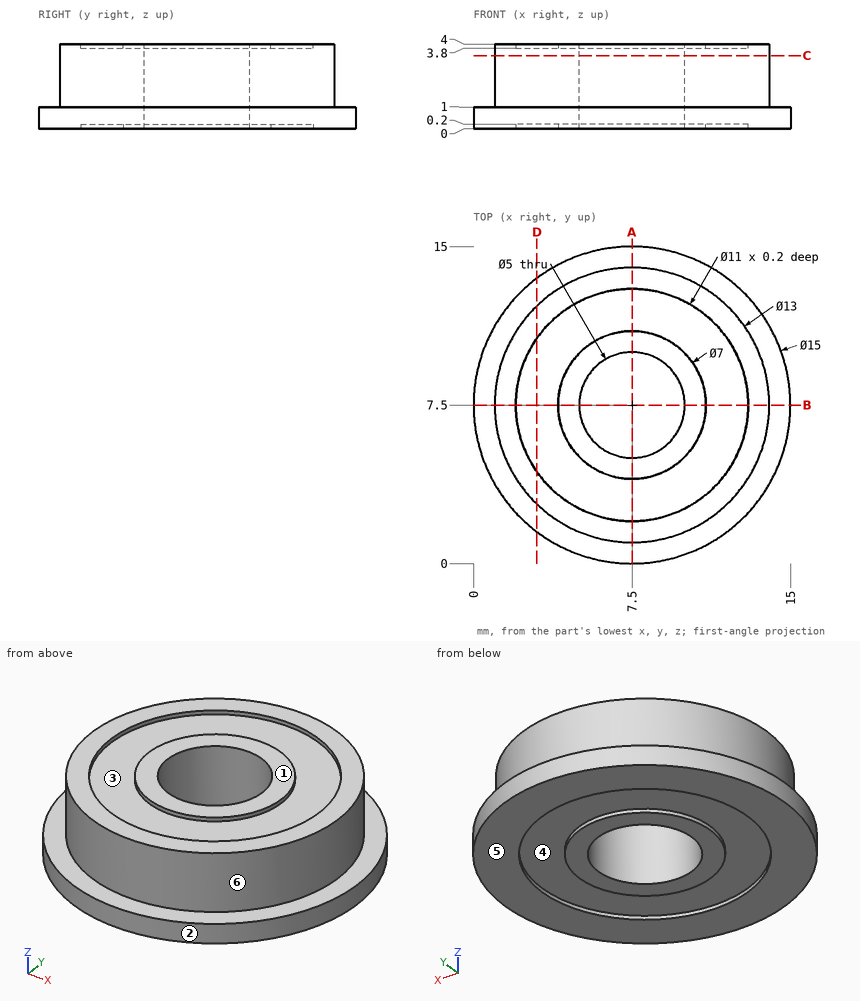
Geometry: see drawing. Coordinates: mm, zero at the bounding-box minimum. A direction names the side the tool comes from. Coordinates: 2 decimals unless noted, no trailing zeros. Loops run counter-clockwise (first coordinate to the right, second up) from the corner with the lowest first, then second, coordinate; pieces in that order, holes last. Notation, with made-up numbers: (12, -29.5) - (60, -29.5) arc R26 ccw to (60, -3.5) - close; hole circle Ø8 at (-9.5, 75). An arc over 180 degrees is marked (long way). Answer in a Markdown table with one row per item.
(1) Cut plane A-A on x = 7.5. Output: boundary loops of the cut face in (y, z), plus the area to 3 significant figures.
Model answer:
| item | result |
|---|---|
| outline | (0, 0) - (2, 0) - (2, 0.2) - (4, 0.2) - (4, 0) - (5, 0) - (5, 4) - (4, 4) - (4, 3.8) - (2, 3.8) - (2, 4) - (1, 4) - (1, 1) - (0, 1) - close; (10, 0) - (11, 0) - (11, 0.2) - (13, 0.2) - (13, 0) - (15, 0) - (15, 1) - (14, 1) - (14, 4) - (13, 4) - (13, 3.8) - (11, 3.8) - (11, 4) - (10, 4) - close |
| area | 32.4 mm² |
(2) Cut plane C-C on z = 3.45. Output: boundary loops of the cut face in (x, y), plus the area to 3 significant figures.
Model answer:
| item | result |
|---|---|
| outline | circle Ø13 at (7.5, 7.5); hole circle Ø5 at (7.5, 7.5) |
| area | 113 mm² |
(3) Pin query (flat end, axial travel): P1, Ø8, axis at x = 3, y = 13, coming from the +Z side; P2, Ø1, axis at x = 10.5, z = 3, coming from the -Y side. Return the tip coordinate at first contact, or that it passes through.
Model answer:
| item | result |
|---|---|
| P1 | stops at z = 4 |
| P2 | stops at y = 1.5 |
(4) Set-up query: the marked faces 4, 5 and 6. Return all of +Z, -Z, +X, -X, +Y, -Y with unobstructed straight access to the full face (end or side cutting, diameter ignored); none if empty.
Model answer:
| item | result |
|---|---|
| face 4 | -Z |
| face 5 | -Z, +X, -X, +Y, -Y |
| face 6 | +Z |
(5) Mould query, pull axis Y, two halves, no side actions, for the marked faces 1, 2 and 3. Classes: pulls with the +Y half, pulls with the -Y half, needs draft (parallel to the pull), parting line crosses it, or undercut.
Model answer:
| item | result |
|---|---|
| face 1 | needs draft |
| face 2 | parting line crosses it |
| face 3 | undercut |
(6) Cut plane D-D on x = 3. Output: boundary loops of the cut face in (y, z).
Model answer:
| item | result |
|---|---|
| outline | (1.5, 0) - (4.34, 0) - (4.34, 0.2) - (10.66, 0.2) - (10.66, 0) - (13.5, 0) - (13.5, 1) - (12.19, 1) - (12.19, 4) - (10.66, 4) - (10.66, 3.8) - (4.34, 3.8) - (4.34, 4) - (2.81, 4) - (2.81, 1) - (1.5, 1) - close |
(7) Material intervals for L1, parallel to Y at x = 7.5, z = 0.15; L2, parallel to Y at x = 7.5, z = 3.9; L3, parallel to Y at x = 7.5, z = 2.1, sorted ascending. Write a range as from..to.
Model answer:
| item | result |
|---|---|
| L1 | y = 0..2, 4..5, 10..11, 13..15 |
| L2 | y = 1..2, 4..5, 10..11, 13..14 |
| L3 | y = 1..5, 10..14 |
